Verification items for the finished model (mm, model axes). A direction names the side the tool comes from. Round coordinates to 2 decimals unless told otherwise and drop trailing zeros. Write each loop counter-clockwise with the first axis right and the second up, starting at its lowest first coordinate (ties: lowest second). Pieces come first, ordered by that corner, then holes. Notation, with made-up numbers: M 19.5,70.5 L 33.5,70.5 A27 cw 33.5,101.5 Z; hole C -8.75,-34 d3. An arc over 180 degrees is marked long. One line per question, with ' | ' between items. Start each with the question number.
Q1. Release check for a two-part mould opening along Z. For faces 6 (the face through (73, 1, 0)), 7 (the face through (-0.62, 1.52, 27)), 8 (the face through (-1, 2, -4.7)) record: released by +Z, released by -Z, zero draft, split by the parting line, or undercut.
Q2. Thickness scan on line 1 along X through (y, z) = (2, 25.5); line 2 along X through (y, z) = (1.7, 11); line 3 along Z through (x, y) = (67, 2.2). Record the ranges inside material, lowest first. Write a range as from..to.
Q3. Cross-section at A-A (z = 12.5). Record the boundary of the cut face in (x, y), then the cut area to 3 significant figures.
Q4. Cross-section at B-B (x = 0). Record the boundary of the cut face in (y, z).
Q5. Cross-section at C-C (y = 2.2). Record the boundary of the cut face in (x, z).
Q6. Tool access check on faces 1 (the face through (-48, 2, 6)), 2 (the face through (73, 1, 25)), 3 (the face through (-1, 0, 13)), 4 (the face through (71, 2, 19.5)), 5 (the face through (-70, 2, 12)). Record the directions out of +Z, -Z, +X, -X, +Y, -Y that give a thin tool (end or side, any length) a straight path to the whole face; none if there is none.
Q7. Gauge pin test, flat ends, axial feed: pin 1 (1.9 mm diameter, centred on x = 0, z = 25.5, fed in from -Y); pin 2 (1.5 mm diameter, centred on y = 1.5, z = 9, fed in from -X). Record the tip position at first contact, or that the pin passes through.
Q8. Cross-section at D-D (z = 25.5). Record the boundary of the cut face in (x, y), then the cut area to 3 significant figures.
from build123d import *

# Parameters (mm, degrees)
SKETCH1_W           = 146
SKETCH1_H           = 61
BOSS_EXTRUDE1_DEPTH = 3
SKETCH2_R           = 1.621357424
SKETCH2_R_2         = 1.718635432
SKETCH2_W           = 3
SKETCH2_H           = 15
SKETCH2_W_2         = 15
SKETCH2_H_2         = 12
SKETCH2_W_3         = 30
SKETCH2_H_3         = 3
CUT_EXTRUDE1_DEPTH  = 10
SKETCH3_W           = 146
SKETCH3_H           = 25.8
CUT_EXTRUDE2_DEPTH  = 10


with BuildPart() as part:
    # Sketch1 → Boss-Extrude1 (new body)
    with BuildSketch(Plane(origin=(0, 0, 0), x_dir=(1, 0, 0), z_dir=(0, 1, 0))):
        Rectangle(SKETCH1_W, SKETCH1_H)
    extrude(amount=BOSS_EXTRUDE1_DEPTH)

    # Sketch2 → Cut-Extrude1 (cut)
    with BuildSketch(Plane(origin=(0, 3, 0), x_dir=(1, 0, 0), z_dir=(0, 1, 0))):
        with Locations(Location((0, -25.5, 0), (0, 0, 270))):
            Circle(SKETCH2_R)
        with Locations(Location((67, -25.5, 0), (0, 0, 270))):
            Circle(SKETCH2_R_2)
        with Locations((-71.5, -12)):
            Rectangle(SKETCH2_W, SKETCH2_H)
        with Locations((71.5, 13)):
            Rectangle(SKETCH2_W, SKETCH2_H)
        with Locations((71.5, -12)):
            Rectangle(SKETCH2_W, SKETCH2_H)
        with Locations((-71.5, 13)):
            Rectangle(SKETCH2_W, SKETCH2_H)
        with Locations((-47.5, -12)):
            Rectangle(SKETCH2_W_2, SKETCH2_H_2)
        with Locations((-28, 29)):
            Rectangle(SKETCH2_W_3, SKETCH2_H_3)
        with Locations((28, 29)):
            Rectangle(SKETCH2_W_3, SKETCH2_H_3)
    extrude(amount=-CUT_EXTRUDE1_DEPTH, mode=Mode.SUBTRACT)

    # Sketch3 → Cut-Extrude2 (cut)
    with BuildSketch(Plane(origin=(0, 3, 0), x_dir=(1, 0, 0), z_dir=(0, 1, 0))):
        with Locations((0, 17.6)):
            Rectangle(SKETCH3_W, SKETCH3_H)
    extrude(amount=-CUT_EXTRUDE2_DEPTH, mode=Mode.SUBTRACT)


solid = part.part
Determined:
1) face 6: zero draft | face 7: undercut | face 8: released by -Z
2) line 1: x = -73..-1.62, 1.62..65.28, 68.72..73 | line 2: x = -70..-55, -40..70 | line 3: z = -4.7..23.78, 27.22..30.5
3) outline: M -70,0 L -55,0 L -55,3 L -70,3 Z; M -40,0 L 70,0 L 70,3 L -40,3 Z | area: 375 mm²
4) outline: M 0,-4.7 L 3,-4.7 L 3,23.88 L 0,23.88 Z; M 0,27.12 L 3,27.12 L 3,30.5 L 0,30.5 Z
5) outline: M -73,-4.7 L 73,-4.7 L 73,4.5 L 70,4.5 L 70,19.5 L 73,19.5 L 73,30.5 L -73,30.5 L -73,19.5 L -70,19.5 L -70,4.5 L -73,4.5 Z; hole M -55,6 L -40,6 L -40,18 L -55,18 Z; hole C 0,25.5 d3.24; hole C 67,25.5 d3.44
6) face 1: +Y, -Y | face 2: +Z, -Z, +X, +Y, -Y | face 3: +Z, -Z, +X, -X, -Y | face 4: +X, +Y, -Y | face 5: -X, +Y, -Y
7) pin 1: passes through | pin 2: stops at x = -70
8) outline: M -73,0 L -1.62,0 L -1.62,3 L -73,3 Z; M 1.62,0 L 65.28,0 L 65.28,3 L 1.62,3 Z; M 68.72,0 L 73,0 L 73,3 L 68.72,3 Z | area: 418 mm²
